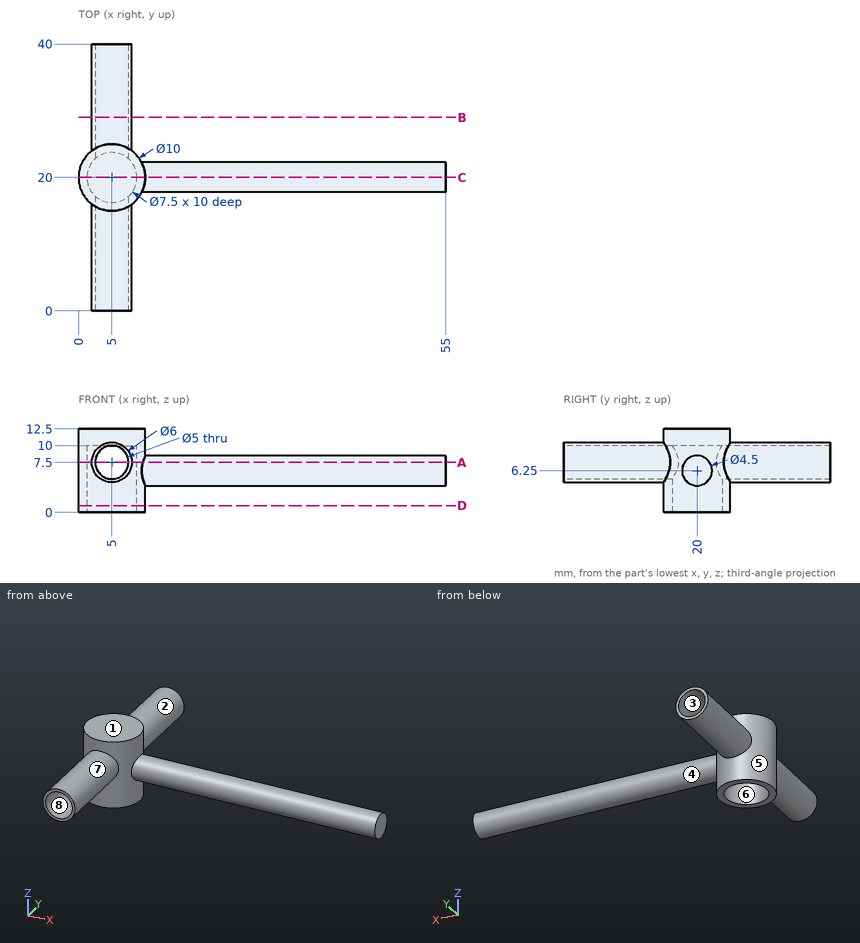
Geometry: see drawing. Coordinates: mm, zero at the bounding-box minimum. A direction names the side the tool comes from. Give positions to 0.01 mm unless a question says otherwise; leave off trailing zeros. Write each loop counter-clockwise with the first axis right and the second up, starting at its lowest first coordinate (ties: lowest second). Pieces come first, ordered by that corner, then holes. Notation, with made-up numbers: (14.25, 11.5) - (21.25, 11.5) arc R33 cw to (21.25, 45.5) - close; hole circle Ø11 at (48.5, 52.5). An arc over 180 degrees is marked (long way). Return JSON: item names as keys, results as strings. Group by question number.
1) Section B-B on y = 29. Return the cut outline in (x, z).
2) First-contact query: P1, Ø3, axis at y = 4.5, z = 3.5, coming from the +X side; P2, Ø2, axis at y = 22.5, z = 3.5, coming from the +X side; P3, Ø10, axis at x = 15.5, y = 20.5, coming from the +Z side. Flat tips, straight axial feed; report the tip coordinate or a pass-through.
3) Mould query, pull axis Z, two halves, no side actions, for the marked faces 1, 2 and 3. Classes: released by +Z, released by -Z, zero draft, split by the parting line, or undercut.
4) Line query: line 1 (X direction, y = 7.5, z = 7.25); line 2 (Z direction, x = 5, y = 33.5); line 3 (X direction, y = 13, z = 8.5). Output: solid intervals per line, ascending.
5) Section A-A on z = 7.5. Return the cut outline in (x, y).
6) Section D-D on z = 1. Return the cut outline in (x, y), plus the area to 3 significant figures.
7) Set-up query: the marked faces 4, 5, 6, 7 and 8. Return all of +Z, -Z, +X, -X, +Y, -Y with unobstructed straight access to the full face (end or side cutting, diameter ignored); none if empty.
8) Section C-C on y = 20. Return the cut outline in (x, z), plus the area to 4 significant figures.
Filled in:
{
 "1": {"outline": "circle Ø6 at (5, 7.5); hole circle Ø5 at (5, 7.5)"},
 "2": {"P1": "stops at x = 6.66", "P2": "stops at x = 9.77", "P3": "stops at z = 8.5"},
 "3": {"face 1": "released by +Z", "face 2": "split by the parting line", "face 3": "undercut"},
 "4": {"line 1": "x = 2.01 to 2.51, 7.49 to 7.99", "line 2": "z = 4.5 to 5, 10 to 10.5", "line 3": "x = 2.17 to 2.71, 7.29 to 7.83"},
 "5": {"outline": "(2, 0) - (2.5, 0) - (2.5, 17.2) arc R3.75 cw to (2.5, 22.8) - (2.5, 40) - (2, 40) - (2, 24) arc R5 ccw to (2, 16) - close; (7.5, 0) - (8, 0) - (8, 16) arc R5 ccw to (9.64, 18.13) - (55, 18.13) - (55, 21.87) - (9.64, 21.87) arc R5 ccw to (8, 24) - (8, 40) - (7.5, 40) - (7.5, 22.8) arc R3.75 cw to (7.5, 17.2) - close"},
 "6": {"outline": "circle Ø10 at (5, 20); hole circle Ø7.5 at (5, 20)", "area": "34.4 mm^2"},
 "7": {"face 4": "+X", "face 5": "none", "face 6": "-Z", "face 7": "-Y", "face 8": "+Y, -Y"},
 "8": {"outline": "(0, 0) - (1.25, 0) - (1.25, 10) - (8.75, 10) - (8.75, 0) - (10, 0) - (10, 4) - (55, 4) - (55, 8.5) - (10, 8.5) - (10, 12.5) - (0, 12.5) - close", "area": "252.5 mm^2"}
}
